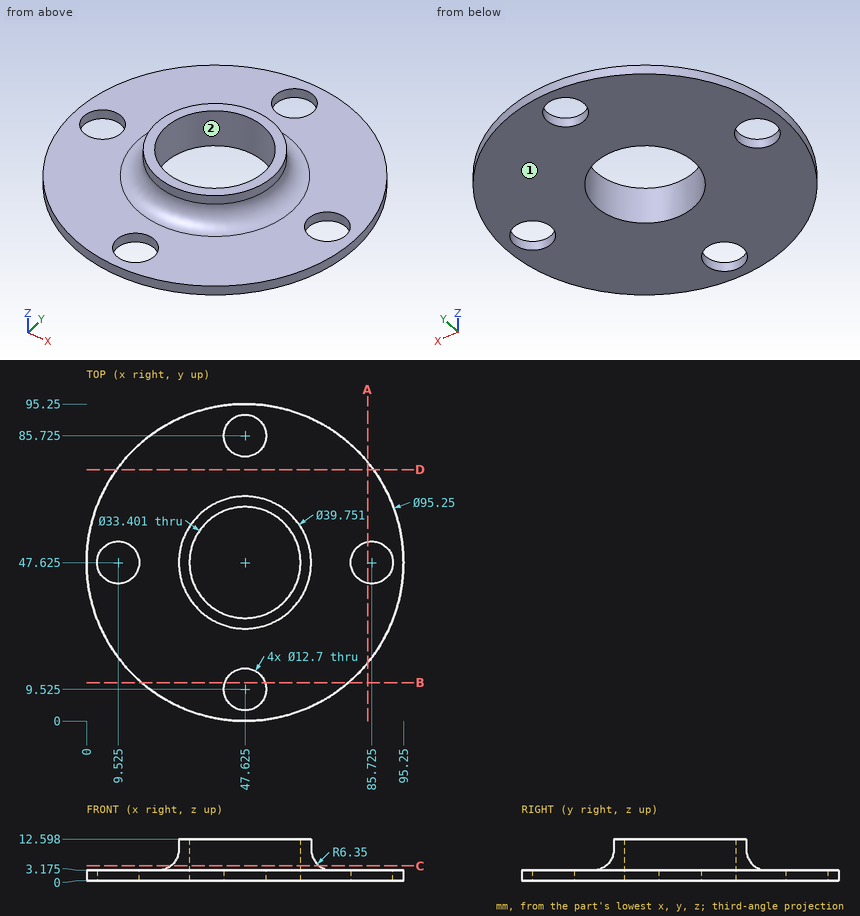
Drawing for the job (mm, zero at the part's lowest x, y, z). Round coordinates to 2 decimals unless told otherwise and drop trailing zeros. Write each loop counter-clockwise with the first axis right and the second up, starting at its lowest first coordinate (ties: lowest second). Pieces come first, ordered by that corner, then holes. Notation, with made-up numbers: M 82.25,26 L 117.25,26 A25 cw 117.25,62 Z; hole C 24.25,84 d2. An arc over 180 degrees is marked long. Answer as a JSON object with one key per item and string values. Group by question number.
(1) Flat gauge pins, fed straight in: pin 1 (2 mm diameter, centred on y = 30.5, z = 3.5, fed in from +X); pin 2 (16.5 mm diameter, centred on x = 47.625, y = 85.725, fed in from +Z) (3 decimals); pin 3 (7.5 mm diameter, centred on x = 9.525, y = 47.625, fed in from +Z); pin 4 (4 mm diameter, centred on x = 53.5, y = 70, fed in from +Z). Where does each tip first touch, or does it go through?
(2) Drill centre lines: L1, parallel to X at y = 48, z = 1.5; L2, parallel to X at y = 51.5, z = 2.5 (1 decimal); L3, parallel to Z at x = 39, y = 76 (1 decimal). Where is each one in solid material? Low to high.
(3) Cut at A-A (x = 84.5). Give the cut face in (y, z) (1 decimal).
(4) Mould opens along Y. For the marked faces 1 and 2 say: pulls with the +Y half, pulls with the -Y half, needs draft (parallel to the pull), parting line crosses it, or undercut.
(5) Cut at B-B (y = 11.5). Give the cut face in (x, z) (1 decimal), and give its area (3 significant figures).
(6) Cut at D-D (y = 75.5). Give the cut face in (x, z) (1 decimal).
(7) Cut at C-C (z = 4.5). Give the cut face in (x, y) (1 decimal), and give its area (3 significant figures).
Responses:
{
 "1": {"pin 1": "stops at x = 92.42", "pin 2": "stops at z = 3.175", "pin 3": "passes through", "pin 4": "stops at z = 5.73"},
 "2": {"L1": "x = 0 to 3.19, 15.86 to 30.93, 64.32 to 79.39, 92.06 to 95.25", "L2": "x = 0.2 to 4.5, 14.6 to 31.4, 63.9 to 80.7, 90.8 to 95.1", "L3": "z = 0 to 3.2"},
 "3": {"outline": "M 17.5,0 L 41.4,0 L 41.4,3.2 L 17.5,3.2 Z; M 53.9,0 L 77.8,0 L 77.8,3.2 L 53.9,3.2 Z"},
 "4": {"face 1": "needs draft", "face 2": "undercut"},
 "5": {"outline": "M 16.6,0 L 41.6,0 L 41.6,3.2 L 16.6,3.2 Z; M 53.7,0 L 78.7,0 L 78.7,3.2 L 53.7,3.2 Z", "area": "159 mm2"},
 "6": {"outline": "M 9,0 L 86.2,0 L 86.2,3.2 L 9,3.2 Z"},
 "7": {"outline": "C 47.6,47.6 d44.7; hole C 47.6,47.6 d33.4", "area": "692 mm2"}
}
